Study the drawing (mm; zero at the part's minimum x, y, z) and answer. Give positions to 0.01 mm unless a question says otherwise; leave off trailing zeros. Loops run counter-clockwise (first coordinate to the right, second up) from the corner with the lowest first, then second, coordinate; pieces in that order, holes last. Notation, with made-up numbers: M 31.25,44 L 35.25,44 A28 cw 35.25,71 Z; hole C 9.5,8.5 d1. An arc over 180 degrees is marked long. Return JSON: item names as keys, results as strings.
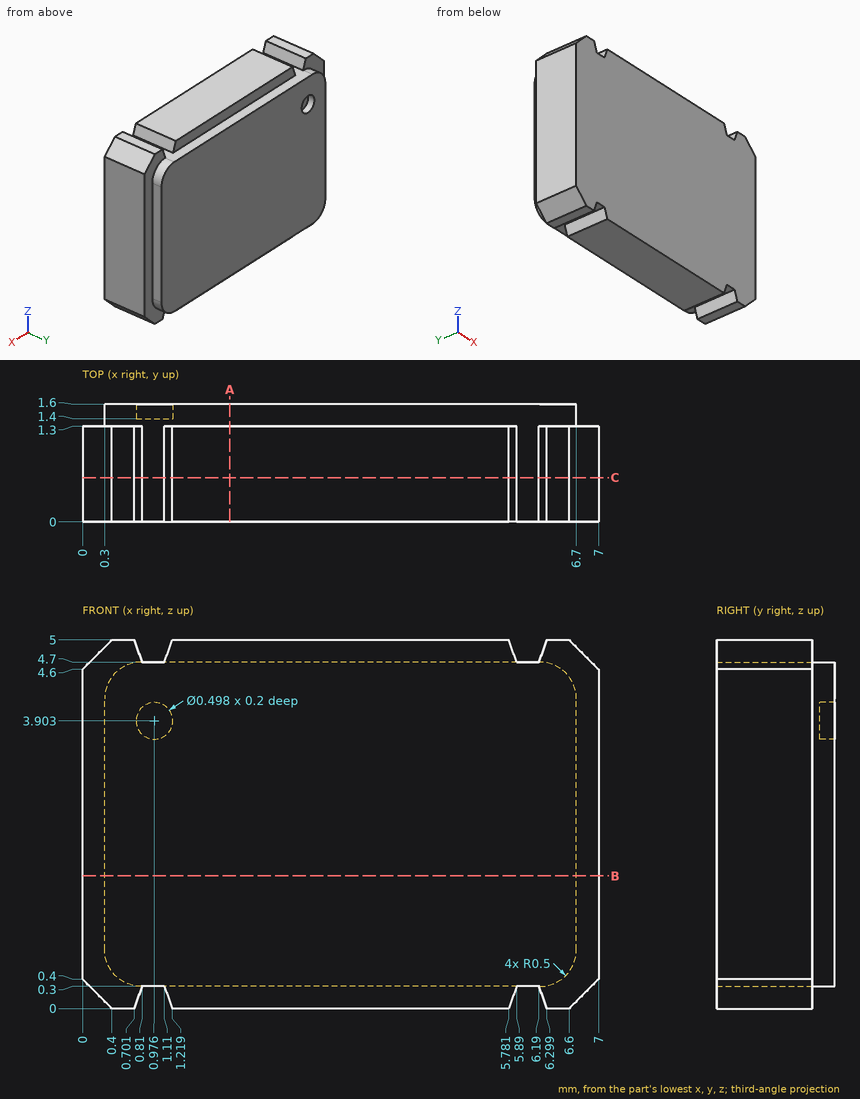
(1) The part is cut by section A-A (x = 2). Determine the outline of the cut face in (y, z).
Values follow:
{"outline": "M 0,0 L 1.3,0 L 1.3,0.3 L 1.6,0.3 L 1.6,4.7 L 1.3,4.7 L 1.3,5 L 0,5 Z"}
(2) Straight lines are drawn through the part: line 1 along Y through (x, z) = (6.75, 4.7); line 2 along Z through (x, y) = (5.75, 1.5); line 3 along X through (y, z) = (1.5, 3.45). For each, find the intervals that lie inside material, in ascending order.
Values follow:
{"line 1": "0 to 1.3", "line 2": "0.3 to 4.7", "line 3": "0.3 to 6.7"}
(3) The part is cut by section C-C (y = 0.6). Determine the outline of the cut face in (x, z).
Values follow:
{"outline": "M 0,0.4 L 0.4,0 L 0.7,0 L 0.81,0.3 L 1.11,0.3 L 1.22,0 L 5.78,0 L 5.89,0.3 L 6.19,0.3 L 6.3,0 L 6.6,0 L 7,0.4 L 7,4.6 L 6.6,5 L 6.3,5 L 6.19,4.7 L 5.89,4.7 L 5.78,5 L 1.22,5 L 1.11,4.7 L 0.81,4.7 L 0.7,5 L 0.4,5 L 0,4.6 Z"}
(4) The part is cut by section B-B (z = 1.8). Determine the outline of the cut face in (x, y), and give its area (3 significant figures).
Values follow:
{"outline": "M 0,0 L 7,0 L 7,1.3 L 6.7,1.3 L 6.7,1.6 L 0.3,1.6 L 0.3,1.3 L 0,1.3 Z", "area": "11.0 mm²"}
